For this review, take the finished solid that the model builds, in its own axes (mm). A direction names the side the tool comes from. Round coordinates to 2 decimals unless told otherwise and drop trailing zeros. Write each loop counter-clockwise with the first axis right and the second up, starting at its lowest first coordinate (ties: lowest second). Pieces come first, ordered by that corner, then holes. Notation, with made-up numbers: (19.5, 5) -> (52.5, 5) arc R7 cw to (52.5, 11) -> close; hole circle Ø5 at (31, 87). An arc over 180 degrees is marked (long way). Answer in a Markdown table with one row per item.
from build123d import *

# Parameters (mm, degrees)
SKETCH1_R           = 18.5
BOSS_EXTRUDE1_DEPTH = 23
SKETCH2_R           = 16.5
BOSS_EXTRUDE2_DEPTH = 23
SKETCH3_R           = 6
BOSS_EXTRUDE3_DEPTH = 6
SKETCH4_R           = 3
BOSS_EXTRUDE4_DEPTH = 12
SKETCH5_W           = 6
SKETCH5_H           = 11.5
CUT_EXTRUDE1_DEPTH  = 12
CIRPATTERN1_COUNT   = 6
SKETCH9_R           = 16.45
BOSS_EXTRUDE5_DEPTH = 9


with BuildPart() as part:
    # Sketch1 → Boss-Extrude1 (new body)
    with BuildSketch(Plane.XY):
        Circle(SKETCH1_R)
    extrude(amount=BOSS_EXTRUDE1_DEPTH)

    # Sketch2 → Boss-Extrude2 (add)
    with BuildSketch(Plane.XY.offset(23)):
        Circle(SKETCH2_R)
    extrude(amount=BOSS_EXTRUDE2_DEPTH)

    # Sketch3 → Boss-Extrude3 (add)
    with BuildSketch(Plane(origin=(0, 0, 0), x_dir=(-1, 0, 0), z_dir=(0, 0, -1))):
        with Locations(Location((0, 7, 0), (0, 0, 180))):
            Circle(SKETCH3_R)
    extrude(amount=BOSS_EXTRUDE3_DEPTH)

    # Sketch4 → Boss-Extrude4 (add)
    with BuildSketch(Plane(origin=(0, 0, -6), x_dir=(-1, 0, 0), z_dir=(0, 0, -1))):
        with Locations((0, 7)):
            Circle(SKETCH4_R)
    extrude(amount=BOSS_EXTRUDE4_DEPTH)

    # Sketch5 → Cut-Extrude1 (cut)
    with BuildSketch(Plane(origin=(0, 9.5, 0), x_dir=(1, 0, 0), z_dir=(0, 1, 0))):
        with Locations((0, 12.25)):
            Rectangle(SKETCH5_W, SKETCH5_H)
    extrude(amount=CUT_EXTRUDE1_DEPTH, mode=Mode.SUBTRACT)

    # Sketch8 → M3 Tapped Hole1 (revolve, cut)
    with BuildSketch(Plane.YZ.offset(15.5)):
        Polygon((0, 0), (0, 5.751075774), (1.25, 5), (1.25, 0), align=None)
    m3_tapped_hole1 = revolve(axis=Axis((15.5, 0, -6.35), (0, 0, 1)), mode=Mode.SUBTRACT)

    # CirPattern1: M3 Tapped Hole1 ×6 about axis
    cirpattern1_axis = Axis((0, 0, 0), (0, 0, 1))
    for i in range(1, CIRPATTERN1_COUNT):
        add(m3_tapped_hole1.rotate(cirpattern1_axis, i * 360 / CIRPATTERN1_COUNT), mode=Mode.SUBTRACT)

    # Sketch9 → Boss-Extrude5 (add)
    with BuildSketch(Plane.XY.offset(46)):
        Circle(SKETCH9_R)
    extrude(amount=BOSS_EXTRUDE5_DEPTH)


solid = part.part
1) Consider section C-C on z = 47.5. State the section outline as (x, y) points, then the cut area to 3 significant figures.
Solved:
| item | result |
|---|---|
| outline | circle Ø32.9 at (0, 0) |
| area | 850 mm² |
2) Consider section A-A on x = 0. State the section outline as (y, z) points, then the cut area to 3 significant figures.
Solved:
| item | result |
|---|---|
| outline | (-18.5, 0) -> (1, 0) -> (1, -6) -> (4, -6) -> (4, -18) -> (9.5, -18) -> (9.5, -6.5) -> (10, -6.5) -> (10, -6) -> (13, -6) -> (13, 0) -> (18.5, 0) -> (18.5, 23) -> (16.5, 23) -> (16.5, 46) -> (16.45, 46) -> (16.45, 55) -> (-16.45, 55) -> (-16.45, 46) -> (-16.5, 46) -> (-16.5, 23) -> (-18.5, 23) -> close |
| area | 2,040 mm² |
3) Clearance check with flat-ended pins moving along their axes: pin 1 Ø1 at (x, z) = (0, -9.5) entering from +Y; pin 2 Ø6 at (y, z) = (-3.5, 32) entering from +X; pin 3 Ø1.5 at (y, z) = (-3.5, 0) entering from +X; pin 4 Ø5 at (x, y) = (4, 7.5) entering from -Z. State where each tip first meets the part, or that it passes through.
Solved:
| item | result |
|---|---|
| pin 1 | y = 9.5 |
| pin 2 | x = 16.49 |
| pin 3 | x = 18.29 |
| pin 4 | z = -18 |
4) Consider section B-B on y = -6. State the section outline as (x, z) points.
Solved:
| item | result |
|---|---|
| outline | (-17.5, 0) -> (17.5, 0) -> (17.5, 23) -> (15.37, 23) -> (15.37, 46) -> (15.32, 46) -> (15.32, 55) -> (-15.32, 55) -> (-15.32, 46) -> (-15.37, 46) -> (-15.37, 23) -> (-17.5, 23) -> close |
5) For faces 1 (the cylindrical face through (15.24, -6.32, 34.34)), 2 (the cylindrical face through (8.804, 12.751, 2.465)), 3 (the flat face through (0, 7, -18)), list the 3-axis set-ups (+Z, -Z, +X, -X, +Y, -Y) from which the entire face can be reached by the end or side of a thin tool; tool diameter is ignored.
Solved:
| item | result |
|---|---|
| face 1 | +Z |
| face 2 | -Z |
| face 3 | -Z, +X, -X, +Y, -Y |
6) Mouldability with a two-part tool opening along Y and no side actions: class faces 4 (the cylindrical face through (-4.01, -18.06, 11.34)), 5 (the flat face through (-17, 0, 23)), 6 (the conical face through (-15.71, 0.05, 5.62)) as pulls with the +Y half, pulls with the -Y half, needs draft (parallel to the pull), parting line crosses it, or undercut.
Solved:
| item | result |
|---|---|
| face 4 | parting line crosses it |
| face 5 | needs draft |
| face 6 | undercut |
7) For line 1 (Y direction, x = -7, z = 2); line 2 (Z direction, x = -11, y = 0.5); line 3 (Z direction, x = 10.5, y = 13), list the stretches that pass through material, from the lowest coordinate up. Write a range as [from, to].
Solved:
| item | result |
|---|---|
| line 1 | [-17.12, -14.42], [-12.42, 12.42], [14.42, 17.12] |
| line 2 | [0, 55] |
| line 3 | [0, 23] |
8) Consider section D-D on x = -4.5. State the section outline as (y, z) points, then the cut area to 3 significant figures.
Solved:
| item | result |
|---|---|
| outline | (-17.94, 0) -> (3.03, 0) -> (3.03, -6) -> (10.97, -6) -> (10.97, 0) -> (17.94, 0) -> (17.94, 23) -> (15.87, 23) -> (15.87, 46) -> (15.82, 46) -> (15.82, 55) -> (-15.82, 55) -> (-15.82, 46) -> (-15.87, 46) -> (-15.87, 23) -> (-17.94, 23) -> close |
| area | 1,890 mm² |
